Read the model definition and answer for the solid it produces. Units are mm, in the model's axes. Face numbers are marked on the shaded views. A direction names the side the tool comes from. Coordinates: 2 decimals unless noted, no trailing zeros. Loops run counter-clockwise (first coordinate to the right, second up) from the corner with the lowest first, then second, coordinate; pieces in that order, holes last.
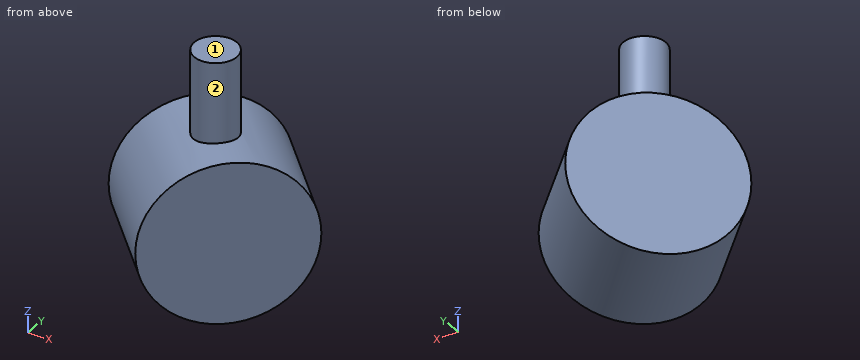
from build123d import *

# Parameters (mm, degrees)
F0_R     = 30
F1_DEPTH = 42
F2_R     = 8
F3_DEPTH = 60
F4_ANGLE = 45


with BuildPart() as f1:
    # F0 (on Front) → F1 (new body)
    with BuildSketch(Plane.XZ):
        Circle(F0_R)
    extrude(amount=F1_DEPTH)

    # F2 (on Top) → F3 (join)
    with BuildSketch(Plane.XY):
        with Locations((0, -21.890162)):
            Circle(F2_R)
    extrude(amount=F3_DEPTH)


with BuildPart() as f1_1:
    # F4: moved
    add(f1.part.rotate(Axis((0, -21.890162, 60), (0, 0, 1)), F4_ANGLE))


solid = f1_1.part
Item 1: A cutting plane is placed at A-A on z = -9. Determine the outline of the cut face in (x, y).
Numbers:
outline: (-35.71, -26.65) - (-6.02, -56.35) - (34.46, -15.87) - (4.76, 13.82) - close
Item 2: Which of the six approach directions +Z, -Z, +X, -X, +Y, -Y give full straight-line access (tool end or side, diameter ignored) to the marked faces 1 and 2?
Numbers:
face 1: +Z, +X, -X, +Y, -Y
face 2: +Z
Item 3: Given pin 1 (1 mm diameter, centred on x = 2, y = -29.5, fed in from -Z); pin 2 (3 mm diameter, centred on x = -22.5, y = -20, fed in from +Z); pin 3 (5 mm diameter, centred on y = -1.5, z = 19.5, fed in from +X), each flat-ended and moving along its own axis, determine where each tip first touches the part or whether it passes through.
Numbers:
pin 1: stops at z = -29.8
pin 2: stops at z = 27
pin 3: stops at x = 15.6
Item 4: Find the intervals of material crossed by line 1 along Z through (x, y) = (9.5, -28); line 2 along X through (y, z) = (-51, -6.5); line 3 along X through (y, z) = (-49.5, -4.5), in increasing order.
Numbers:
line 1: z = -29.9 to 29.9
line 2: x = -12.31 to -0.67
line 3: x = -14.34 to 0.83
